For this review, use the dimensioned drawing (mm, ordinates from the lowest corner) and the shaded views. A direction names the side the tool comes from. Give positions to 0.01 mm unless a question says otherwise; leave off trailing zeros. Write each loop counter-clockwise with the first axis right and the second up, starting at its lowest first coordinate (ties: lowest second). Pieces come first, ordered by that corner, then holes. Notation, with made-up numbers: (-11, 57.25) - (13, 57.25) arc R27 cw to (13, 74.25) - close; hole circle Ø10 at (-6.75, 69). An arc over 180 degrees is marked (long way). One line per question, with ' | ' between items. Start each with the question number.
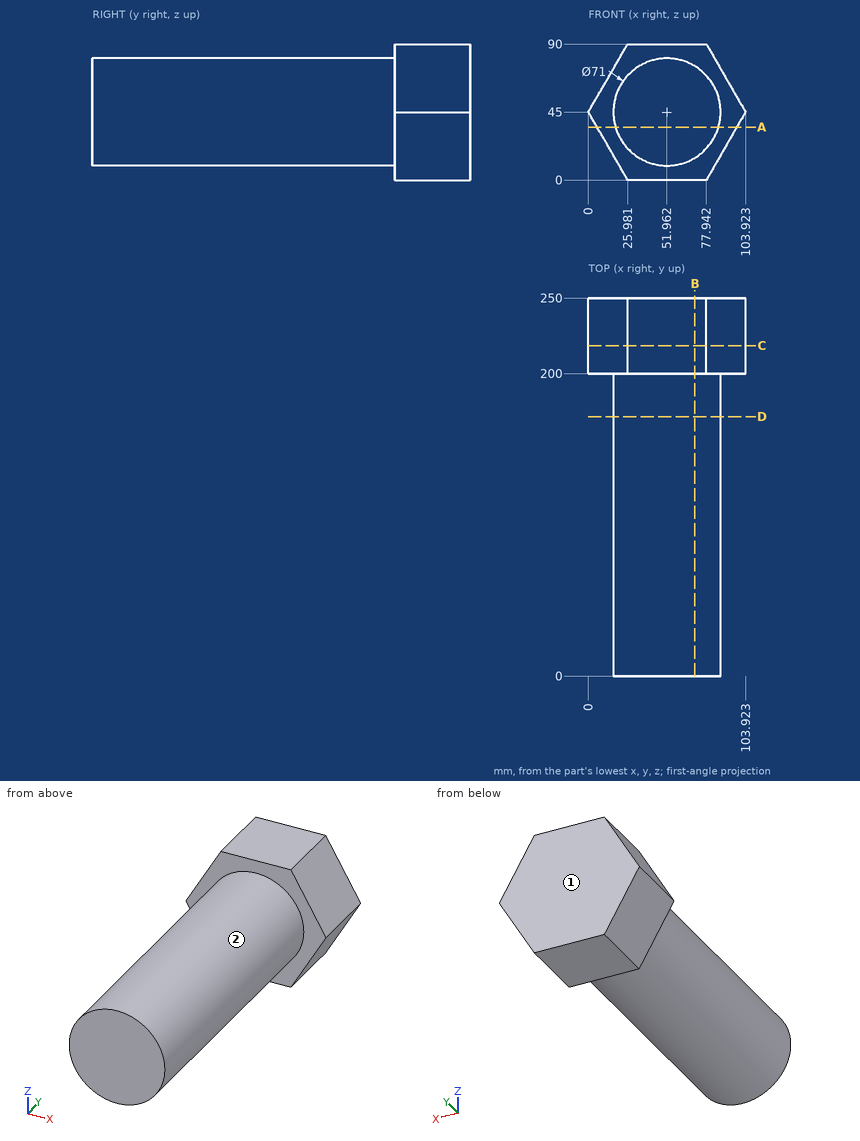
Item 1: Take a section at C-C (y = 218.5). Give the boundary of the cut face in (x, z).
Item 2: Take a section at A-A (z = 35). Give the boundary of the cut face in (x, y).
Item 3: Take a section at B-B (x = 70.5). Give the boundary of the cut face in (y, z) (1 decimal), plus the area to 3 significant figures.
Item 4: Clearance check with flat-ended pins moving along their axes: P1, Ø1.5, axis at x = 78, y = 171, coming from the -Z side (1 decimal); P2, Ø12, axis at y = 150.5, z = 34.5, coming from the -X side; P3, Ø2, axis at x = 29.5, y = 142, coming from the +Z side. State where each tip first meets the part, or that it passes through.
Item 5: Take a section at D-D (y = 171.5). Give the boundary of the cut face in (x, z), plus the area to 3 significant figures.
Item 6: Machinability: for the marked faces 1 and 2, which of the approach directions +Z, -Z, +X, -X, +Y, -Y give a long, thin tool a straight path to every point of the face, cutting with its end or side? Answer none if there is none.
Item 7: For probe 1 along Z at (x, y) = (53, 71) (1 decimal); probe 2 along X at (y, z) = (55.5, 46) (1 decimal); probe 3 along Y at (x, z) = (98, 49), list the stretches that pass through material, from the lowest coordinate up.
Check sheet entries:
1) outline: (0, 45) - (25.98, 0) - (77.94, 0) - (103.92, 45) - (77.94, 90) - (25.98, 90) - close
2) outline: (5.77, 200) - (17.9, 200) - (17.9, 0) - (86.02, 0) - (86.02, 200) - (98.15, 200) - (98.15, 250) - (5.77, 250) - close
3) outline: (0, 14.7) - (200, 14.7) - (200, 0) - (250, 0) - (250, 90) - (200, 90) - (200, 75.3) - (0, 75.3) - close | area: 16,600 mm^2
4) P1: stops at z = 20.1 | P2: stops at x = 16.75 | P3: stops at z = 73.28
5) outline: circle Ø71 at (51.96, 45) | area: 3,960 mm^2
6) face 1: +Z, -Z, +X, -X, +Y | face 2: -Y
7) probe 1: z = 9.5 to 80.5 | probe 2: x = 16.5 to 87.4 | probe 3: y = 200 to 250
